Input: dimensioned drawing with shaded views. Units: mm. Origin: part minimum x, y, z. A direction names the side the tool comes from. Coordinates: 2 decimals unless noted, no trailing zeros. Order: outer loops, then holes, each group sorted by start corner. A loop starts at its lowest first (then second) coordinate and runs counter-clockwise, first axis right, second up. Notation, with made-up numbers: (-19, 43.5) -> (-3, 43.5) arc R14 ccw to (-3, 52.5) -> close; hole circle Ø7 at (42, 76.5). An arc over 180 degrees is marked (long way). Put each result on its own line as item: value.
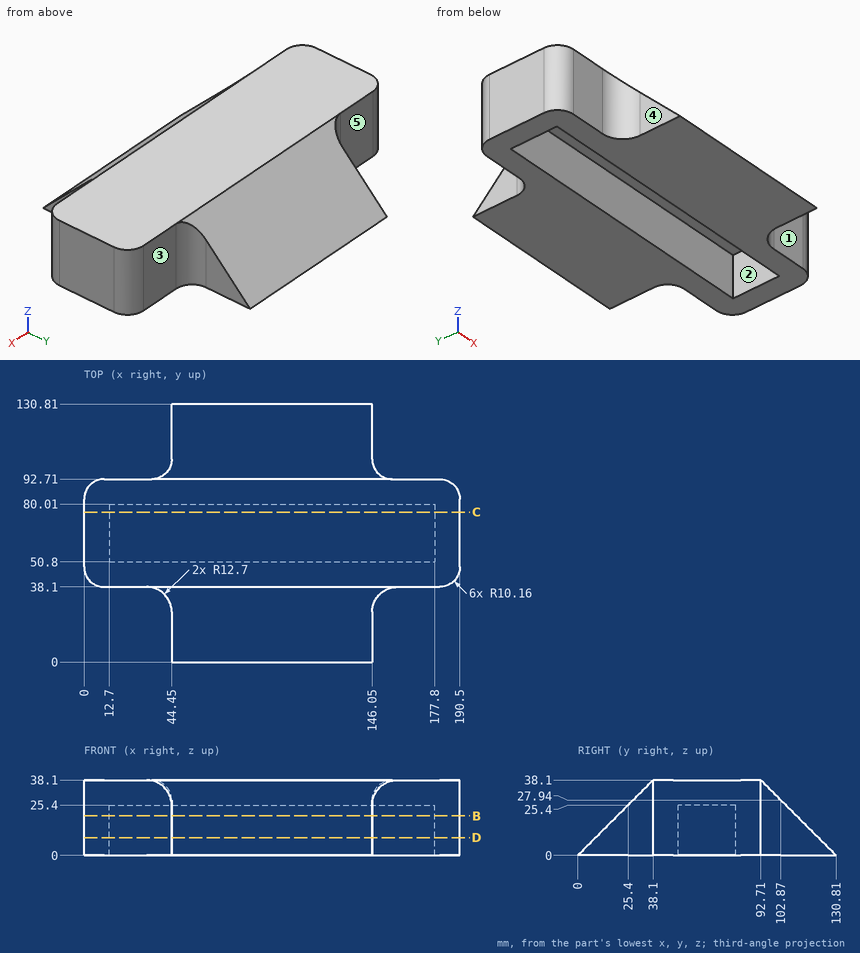
1. First-contact query: pin 1 (1.5 mm diameter, centred on x = 84.5, z = 16, fed in from +Y); pin 2 (4 mm diameter, centred on x = 30.5, z = 9, fed in from +Y); pin 3 (17.5 mm diameter, centred on x = 25, z = 16, fed in from -Y). Flat tips, straight axial feed; report the tip coordinate or a pass-through.
Numbers:
pin 1: stops at y = 115.56
pin 2: stops at y = 92.71
pin 3: stops at y = 37.94
2. Cut plane C-C on y = 76. Output: boundary loops of the cut face in (x, z).
Numbers:
outline: (0, 0) -> (12.7, 0) -> (12.7, 25.4) -> (177.8, 25.4) -> (177.8, 0) -> (190.5, 0) -> (190.5, 38.1) -> (0, 38.1) -> close
3. Cut plane B-B on z = 20. Output: boundary loops of the cut face in (x, y), plus the area to 3 significant figures.
Numbers:
outline: (0, 48.26) arc R10.16 ccw to (10.16, 38.1) -> (31.75, 38.1) arc R12.7 cw to (44.45, 25.4) -> (44.45, 20) -> (146.05, 20) -> (146.05, 25.4) arc R12.7 cw to (158.75, 38.1) -> (180.34, 38.1) arc R10.16 ccw to (190.5, 48.26) -> (190.5, 82.55) arc R10.16 ccw to (180.34, 92.71) -> (156.21, 92.71) arc R10.16 cw to (146.05, 102.87) -> (146.05, 110.81) -> (44.45, 110.81) -> (44.45, 102.87) arc R10.16 cw to (34.29, 92.71) -> (10.16, 92.71) arc R10.16 ccw to (0, 82.55) -> close; hole (12.7, 50.8) -> (177.8, 50.8) -> (177.8, 80.01) -> (12.7, 80.01) -> close
area: 9,280 mm2
4. Cut plane D-D on z = 9. Output: boundary loops of the cut face in (x, y), plus the area to 3 significant figures.
Numbers:
outline: (0, 48.26) arc R10.16 ccw to (10.16, 38.1) -> (31.75, 38.1) arc R12.7 cw to (44.45, 25.4) -> (44.45, 9) -> (146.05, 9) -> (146.05, 25.4) arc R12.7 cw to (158.75, 38.1) -> (180.34, 38.1) arc R10.16 ccw to (190.5, 48.26) -> (190.5, 82.55) arc R10.16 ccw to (180.34, 92.71) -> (156.21, 92.71) arc R10.16 cw to (146.05, 102.87) -> (146.05, 121.81) -> (44.45, 121.81) -> (44.45, 102.87) arc R10.16 cw to (34.29, 92.71) -> (10.16, 92.71) arc R10.16 ccw to (0, 82.55) -> close; hole (12.7, 50.8) -> (177.8, 50.8) -> (177.8, 80.01) -> (12.7, 80.01) -> close
area: 11,500 mm2
5. Set-up query: the marked faces 1, 2, 3, 4 and 5. Return all of +Z, -Z, +X, -X, +Y, -Y with unobstructed straight access to the full face (end or side cutting, diameter ignored); none if empty.
Numbers:
face 1: +Z, -Z, +X, -Y
face 2: -Z
face 3: +Z, -Z, +X, +Y
face 4: +Z, -Z, -X, -Y
face 5: +Z, -Z, -X, +Y
6. Ray query, line 1 along X through (y, z) = (77, 10.5); line 2 along Y through (x, z) = (171, 33); line 3 along Y through (x, z) = (31, 2.5). Return the intervals inside material, ascending.
Numbers:
line 1: x = 0 to 12.7, 177.8 to 190.5
line 2: y = 38.1 to 92.71
line 3: y = 38.1 to 50.8, 80.01 to 92.71
